Geometry: final body of the model. Coordinates: model frame, mm. Give positions to 0.01 mm unless a question says otherwise; leave off trailing zeros. Write each loop counter-clockwise with the first axis right and the second up, starting at its lowest first coordinate (ties: lowest second). Pieces come first, ordered by that corner, then holes. Notation, with made-up numbers: (-6.5, -16.75) -> (45.5, -16.75) arc R24 ccw to (45.5, 22.25) -> close; hole circle Ø7 at (73, 24.25). An arc over 180 degrees is marked (long way). Answer in a Markdown table with one row per item. Add a question column.
Item 1: Section query A-A on y = -12. Output: boundary loops of the cut face in (x, z).
Item 2: First-contact query: P1, Ø3, axis at x = -2.5, y = -7, coming from the -Z side; P2, Ø6, axis at x = 1.5, z = 3, coming from the +Y side; P3, Ø1.5, axis at y = -8.5, z = -1.5, coming from the +X side. Flat tips, straight axial feed; report the tip coordinate or a pass-through.
Item 3: Material intervals for probe 1 along X at (y, z) = (-13.75, -0.25); probe 2 along Y at (x, z) = (0, 4.75); probe 3 along Z at (x, y) = (-1.75, -3), sorted ascending. Write a range as from..to.
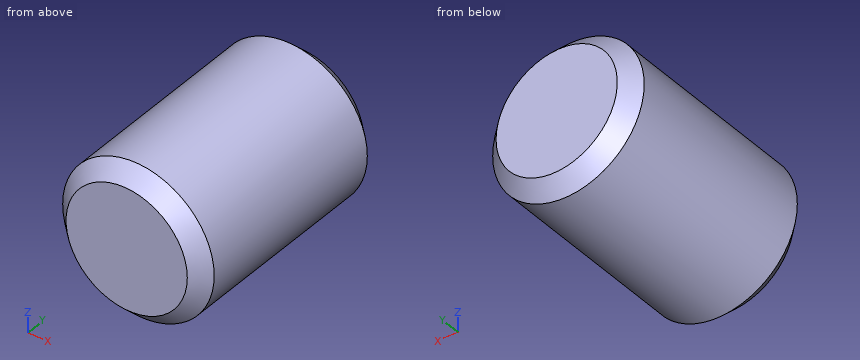
```python
from build123d import *

# Parameters (mm, degrees)
F0_R     = 5
F1_DEPTH = 15
F2_SIZE  = 1
F3_SIZE  = 1


with BuildPart() as f1:
    # F0 (on Front) → F1 (new body)
    with BuildSketch(Plane.XZ):
        Circle(F0_R)
    extrude(amount=F1_DEPTH)

    # F2
    f2_edges = [f1.edges().sort_by_distance(p)[0] for p in [
        (-5, 0, 0),
    ]]
    chamfer(f2_edges, length=F2_SIZE)

    # F3
    f3_edges = [f1.edges().sort_by_distance(p)[0] for p in [
        (-5, -15, 0),
    ]]
    chamfer(f3_edges, length=F3_SIZE)


solid = f1.part
```
Findings below:
| question | item | result |
|---|---|---|
| 1 | outline | circle Ø10 at (0, 0) |
| 2 | P1 | stops at z = -4.9 |
| 2 | P2 | stops at y = 0 |
| 2 | P3 | stops at x = 4.94 |
| 3 | probe 1 | x = -4.99..4.99 |
| 3 | probe 2 | y = -14.25..-0.75 |
| 3 | probe 3 | z = -4.68..4.68 |
